Build history of the part. All positions in model axes, mm. Coordinates: 2 decimals unless noted, no trailing zeros. Loops run counter-clockwise (first coordinate to the right, second up) from the corner with the lowest first, then second, coordinate; pieces in that order, holes last. Notation, with made-up numbers: (40.5, 56) - (86.5, 56) arc R15 ccw to (86.5, 75) - close; hole circle Ø10 at (55.25, 10). An arc over 180 degrees is marked (long way). One line per item, written item: value.
```python
from build123d import *

# Parameters (mm, degrees)
SKETCH_1_W          = 60
SKETCH_1_H          = 60
EXTRUDE_1_DEPTH     = 4
EXTRUDE_2_DEPTH     = 4
SKETCH_3_R          = 16
EXTRUDE_3_DEPTH     = 4
SKETCH_4_R          = 6
CUT_EXTRUDE_1_DEPTH = 133.687643579
SKETCH_5_R          = 1.75
CUT_EXTRUDE_2_DEPTH = 133.687643579
SKETCH_6_R          = 4
CUT_EXTRUDE_3_DEPTH = 133.687643579
SKETCH_7_R          = 1.6
CUT_EXTRUDE_4_DEPTH = 133.687643579
CUT_EXTRUDE_5_DEPTH = 133.687643579
FILLET_1_R          = 5


with BuildPart() as part:
    # 草图1 → 凸台-拉伸1 (new body)
    with BuildSketch(Plane.XY):
        Rectangle(SKETCH_1_W, SKETCH_1_H)
    extrude(amount=EXTRUDE_1_DEPTH)

    # 草图2 → 凸台-拉伸2 (add)
    with BuildSketch(Plane.XY):
        Polygon((18.686292, 30), (72.12484, 83.43854), (83.43854, 72.12484), (30, 18.686292), align=None)
        Polygon((-18.686292, 30), (-72.12484, 83.43854), (-83.43854, 72.12484), (-30, 18.686292), align=None)
        Polygon((-30, -18.686292), (-83.43854, -72.12484), (-72.12484, -83.43854), (-18.686292, -30), align=None)
        Polygon((30, -18.686292), (83.43854, -72.12484), (72.12484, -83.43854), (18.686292, -30), align=None)
    extrude(amount=EXTRUDE_2_DEPTH)

    # 草图3 → 凸台-拉伸3 (add)
    with BuildSketch(Plane.XY):
        with Locations((77.78169, 77.78169)):
            Circle(SKETCH_3_R)
        with Locations((-77.78169, 77.78169)):
            Circle(SKETCH_3_R)
        with Locations((-77.78169, -77.78169)):
            Circle(SKETCH_3_R)
        with Locations((77.78169, -77.78169)):
            Circle(SKETCH_3_R)
    extrude(amount=EXTRUDE_3_DEPTH)

    # 草图4 → 切除-拉伸1 (cut, through all)
    with BuildSketch(Plane.XY):
        Circle(SKETCH_4_R)
    extrude(amount=CUT_EXTRUDE_1_DEPTH, mode=Mode.SUBTRACT)

    # 草图5 → 切除-拉伸2 (cut, through all)
    with BuildSketch(Plane.XY):
        with Locations((15.25, 15.25)):
            Circle(SKETCH_5_R)
        with Locations((-15.25, 15.25)):
            Circle(SKETCH_5_R)
        with Locations((-15.25, -15.25)):
            Circle(SKETCH_5_R)
        with Locations((15.25, -15.25)):
            Circle(SKETCH_5_R)
    extrude(amount=CUT_EXTRUDE_2_DEPTH, mode=Mode.SUBTRACT)

    # 草图6 → 切除-拉伸3 (cut, through all)
    with BuildSketch(Plane.XY):
        with Locations((77.78169, 77.78169)):
            Circle(SKETCH_6_R)
        with Locations((-77.78169, 77.78169)):
            Circle(SKETCH_6_R)
        with Locations((-77.78169, -77.78169)):
            Circle(SKETCH_6_R)
        with Locations((77.78169, -77.78169)):
            Circle(SKETCH_6_R)
    extrude(amount=CUT_EXTRUDE_3_DEPTH, mode=Mode.SUBTRACT)

    # 草图7 → 切除-拉伸4 (cut, through all)
    with BuildSketch(Plane.XY):
        with Locations((87.28169, 77.78169)):
            Circle(SKETCH_7_R)
        with Locations((68.28169, 77.78169)):
            Circle(SKETCH_7_R)
        with Locations((77.78169, 87.28169)):
            Circle(SKETCH_7_R)
        with Locations((77.78169, 68.28169)):
            Circle(SKETCH_7_R)
        with Locations((-87.28169, 77.78169)):
            Circle(SKETCH_7_R)
        with Locations((-68.28169, 77.78169)):
            Circle(SKETCH_7_R)
        with Locations((-77.78169, 87.28169)):
            Circle(SKETCH_7_R)
        with Locations((-77.78169, 68.28169)):
            Circle(SKETCH_7_R)
        with Locations((-87.28169, -77.78169)):
            Circle(SKETCH_7_R)
        with Locations((-68.28169, -77.78169)):
            Circle(SKETCH_7_R)
        with Locations((-77.78169, -87.28169)):
            Circle(SKETCH_7_R)
        with Locations((-77.78169, -68.28169)):
            Circle(SKETCH_7_R)
        with Locations((87.28169, -77.78169)):
            Circle(SKETCH_7_R)
        with Locations((68.28169, -77.78169)):
            Circle(SKETCH_7_R)
        with Locations((77.78169, -87.28169)):
            Circle(SKETCH_7_R)
        with Locations((77.78169, -68.28169)):
            Circle(SKETCH_7_R)
    extrude(amount=CUT_EXTRUDE_4_DEPTH, mode=Mode.SUBTRACT)

    # 草图8 → 切除-拉伸5 (cut, through all)
    with BuildSketch(Plane.XY):
        with BuildLine():
            Line((33.941130344, 29.698489656), (55.154330344, 50.911689656))
            ThreePointArc((55.154330344, 50.911689656), (55.154330344, 55.154330344), (50.911689656, 55.154330344))
            Line((50.911689656, 55.154330344), (29.698489656, 33.941130344))
            ThreePointArc((29.698489656, 33.941130344), (29.698489656, 29.698489656), (33.941130344, 29.698489656))
        make_face()
        with BuildLine():
            Line((-29.698489656, 33.941130344), (-50.911689656, 55.154330344))
            ThreePointArc((-50.911689656, 55.154330344), (-55.154330344, 55.154330344), (-55.154330344, 50.911689656))
            Line((-55.154330344, 50.911689656), (-33.941130344, 29.698489656))
            ThreePointArc((-33.941130344, 29.698489656), (-29.698489656, 29.698489656), (-29.698489656, 33.941130344))
        make_face()
        with BuildLine():
            Line((-33.941130344, -29.698489656), (-55.154330344, -50.911689656))
            ThreePointArc((-55.154330344, -50.911689656), (-55.154330344, -55.154330344), (-50.911689656, -55.154330344))
            Line((-50.911689656, -55.154330344), (-29.698489656, -33.941130344))
            ThreePointArc((-29.698489656, -33.941130344), (-29.698489656, -29.698489656), (-33.941130344, -29.698489656))
        make_face()
        with BuildLine():
            Line((29.698489656, -33.941130344), (50.911689656, -55.154330344))
            ThreePointArc((50.911689656, -55.154330344), (55.154330344, -55.154330344), (55.154330344, -50.911689656))
            Line((55.154330344, -50.911689656), (33.941130344, -29.698489656))
            ThreePointArc((33.941130344, -29.698489656), (29.698489656, -29.698489656), (29.698489656, -33.941130344))
        make_face()
    extrude(amount=CUT_EXTRUDE_5_DEPTH, mode=Mode.SUBTRACT)

    # 圆角1
    fillet_1_edges = [part.edges().sort_by_distance(p)[0] for p in [
        (30, -18.686292, 2),
        (18.686292, -30, 2),
        (-18.686292, -30, 2),
        (-30, -18.686292, 2),
        (-30, 18.686292, 2),
        (-18.686292, 30, 2),
        (18.686292, 30, 2),
        (30, 18.686292, 2),
    ]]
    fillet(fillet_1_edges, radius=FILLET_1_R)


solid = part.part
```
Item 1: Drop flat-ended pins along their axis: P1, Ø1, axis at x = -68.5, z = 2.5, coming from the +Y side; P2, Ø5, axis at x = -77.78, y = 77.78, coming from the +Z side; P3, Ø2, axis at x = -59.5, z = 2, coming from the +Y side. Give the stop position or say it passes through.
Check result:
P1: stops at y = 91.16
P2: passes through
P3: stops at y = 71.81
Item 2: Cut at B-B, the plane x = 41.5. Write the cut outline in (y, z), then the cut area to 3 significant figures.
Check result:
outline: (-52.81, 0) - (-45.74, 0) - (-45.74, 4) - (-52.81, 4) - close; (-37.26, 0) - (-30.19, 0) - (-30.19, 4) - (-37.26, 4) - close; (30.19, 0) - (37.26, 0) - (37.26, 4) - (30.19, 4) - close; (45.74, 0) - (52.81, 0) - (52.81, 4) - (45.74, 4) - close
area: 113 mm^2
Item 3: Cut at D-D, the plane z = 0.85. Give the number of separate pieces and of enclosed holes in the cut face, then the cut area to 3 significant figures.
Check result:
separate pieces: 1
enclosed holes: 29
area: 9,110 mm^2
Item 4: Pull direction Y, two halves, no side cores. Call faces 1 (the face through (0, -30, 2)), 2 (the face through (-55.11, 55.2, 1.97)), 3 (the face through (0, 30, 2)), 4 (the face through (-29.65, -29.75, 1.97)): released by +Y, released by -Y, zero draft, split by the parting line, or undercut.
Check result:
face 1: released by -Y
face 2: undercut
face 3: released by +Y
face 4: undercut
Item 5: Probe probe 1 along Y at (x, z) = (-15.25, 2.1); probe 2 along Y at (x, z) = (32, 0.3); probe 3 along X at (y, z) = (68, 2.2). List the from-to ranges inside material, lowest first. Write a range as from..to.
Check result:
probe 1: y = -30..-17, -13.5..13.5, 17..30
probe 2: y = -43.31..-36.24, -28.83..-20.69, 20.69..28.83, 36.24..43.31
probe 3: x = -90.44..-79.36, -76.21..-56.69, 56.69..76.21, 79.36..90.44
Item 6: Cut at C-C, the plane y = 47. Write the cut outline in (x, z), then the cut area to 3 significant figures.
Check result:
outline: (-58.31, 0) - (-51.24, 0) - (-51.24, 4) - (-58.31, 4) - close; (-42.76, 0) - (-35.69, 0) - (-35.69, 4) - (-42.76, 4) - close; (35.69, 0) - (42.76, 0) - (42.76, 4) - (35.69, 4) - close; (51.24, 0) - (58.31, 0) - (58.31, 4) - (51.24, 4) - close
area: 113 mm^2
Item 7: Cut at A-A, the plane y = 0. Write the cut outline in (x, z), then the cut area to 3 significant figures.
Check result:
outline: (-30, 0) - (-6, 0) - (-6, 4) - (-30, 4) - close; (6, 0) - (30, 0) - (30, 4) - (6, 4) - close
area: 192 mm^2
